Input: part model. Units: mm. Frame: model coordinates. Coordinates: 2 decimals unless noted, no trailing zeros. Loops run counter-clockwise (first coordinate to the right, second up) from the corner with the lowest first, then second, coordinate; pieces in that order, holes last. Notation, with made-up numbers: (25, 25) -> (35, 25) arc R14 cw to (35, 34) -> close; hole circle Ø8 at (61, 86). An arc over 180 degrees is marked (long way). Answer as a JSON object with one key per item and string values.
from build123d import *

# Parameters (mm, degrees)
SKETCH3_R                = 3.175
SKETCH3_R_2              = 1.778
BOSS_EXTRUDE1_DEPTH      = 2.38125
BOSS_EXTRUDE1_DEPTH_BACK = 2.38125
CHAMFER1_SIZE            = 0.1397


with BuildPart() as part:
    # Sketch3 → Boss-Extrude1 (new body, two sides)
    with BuildSketch(Plane.XY) as boss_extrude1_sk:
        Circle(SKETCH3_R)
        Circle(SKETCH3_R_2, mode=Mode.SUBTRACT)
    extrude(amount=BOSS_EXTRUDE1_DEPTH)
    extrude(boss_extrude1_sk.sketch, amount=-BOSS_EXTRUDE1_DEPTH_BACK)

    # Chamfer1
    chamfer1_edges = [part.edges().sort_by_distance(p)[0] for p in [
        (-3.175, 0, -2.38125),
        (-1.778, 0, -2.38125),
        (-3.175, 0, 2.38125),
        (-1.778, 0, 2.38125),
    ]]
    chamfer(chamfer1_edges, length=CHAMFER1_SIZE)


solid = part.part
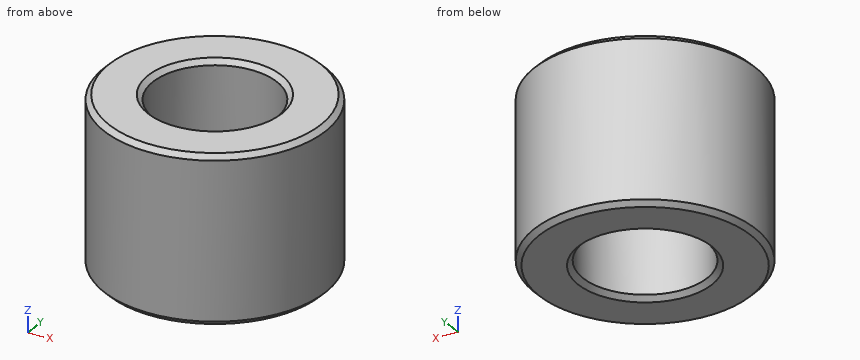
1. Section query C-C (z = -0.15). Return loops of the section in (x, y) (3 decimals), plus the area to 3 significant figures.
Reply:
{"outline": "circle Ø6.35 at (0, 0); hole circle Ø3.556 at (0, 0)", "area": "21.7 mm2"}
2. Section query A-A (x = 0). Return loops of the section in (y, z) (3 decimals), plus the area to 3 significant figures.
Reply:
{"outline": "(-3.175, -2.242) -> (-3.035, -2.381) -> (-1.918, -2.381) -> (-1.778, -2.242) -> (-1.778, 2.242) -> (-1.918, 2.381) -> (-3.035, 2.381) -> (-3.175, 2.242) -> close; (1.778, -2.242) -> (1.918, -2.381) -> (3.035, -2.381) -> (3.175, -2.242) -> (3.175, 2.242) -> (3.035, 2.381) -> (1.918, 2.381) -> (1.778, 2.242) -> close", "area": "13.2 mm2"}
3. Line query: line 1 along Y through (x, z) = (0, 0.95) (3 decimals); line 2 along X through (y, z) = (-1.5, -1.7); line 3 along X through (y, z) = (0.5, 0.45). Output: solid intervals per line, ascending.
Reply:
{"line 1": "y = -3.175 to -1.778, 1.778 to 3.175", "line 2": "x = -2.8 to -0.95, 0.95 to 2.8", "line 3": "x = -3.14 to -1.71, 1.71 to 3.14"}
4. Pin query (flat end, axial travel): P1, Ø1, axis at x = -1.5, z = 0.5, coming from the -Y side; P2, Ø3, axis at x = 0, y = 0, coming from the +Z side. Return the tip coordinate at first contact, or that it passes through.
Reply:
{"P1": "stops at y = -3.01", "P2": "passes through"}
